Source: three-view drawing plus pictorial views. Frame: mm from the lowest corner of the part. Round coordinates to 2 decimals unless told otherwise and drop trailing zeros. Loops run counter-clockwise (first coordinate to the right, second up) from the corner with the lowest first, then second, coordinate; pieces in that order, holes last. Notation, with made-up numbers: (45.5, 85.25) -> (76.5, 85.25) arc R20 ccw to (76.5, 118.25) -> close; hole circle Ø7 at (46.25, -20). An arc over 180 degrees is marked (long way). Answer as a JSON object with one key per item and string values. Group by question number.
Item 1: Section query D-D on y = 3.3. Return loops of the section in (x, z).
Item 2: Section query C-C on x = 24. Return loops of the section in (y, z), and give its area (3 significant figures).
Item 3: Section query A-A on x = 70.5. Return loops of the section in (y, z).
Item 4: Section query B-B on z = 44. Return loops of the section in (x, y).
Item 5: Pin query (flat end, axial travel): pin 1 (10 mm diameter, centred on x = 38, z = 23.5, fed in from +Y); pin 2 (5.5 mm diameter, centred on x = 4, z = 44, fed in from -Y); pin 3 (0.9 mm diameter, centred on y = 3.5, z = 35, fed in from -X); pin 4 (1 mm diameter, centred on y = 3.5, z = 36, fed in from +X). Return the tip coordinate at first contact, or that it passes through.
Item 6: Material intervals for line 1 (X direction, y = 1.15, z = 44); line 2 (Y direction, x = 42.5, z = 30); line 3 (X direction, y = 3, z = 13), sorted ascending. Write a range as [from, to].
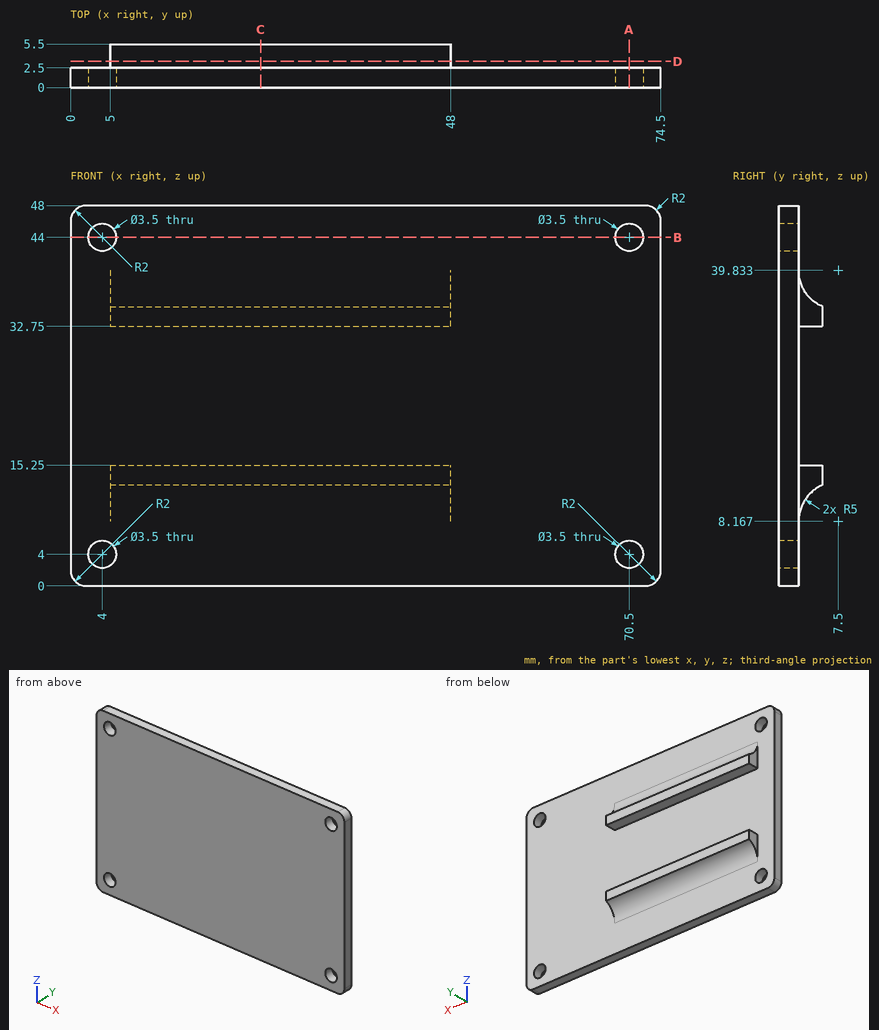
Solved:
{
 "1": {"outline": "(5, 10.88) -> (48, 10.88) -> (48, 15.25) -> (5, 15.25) -> close; (5, 32.75) -> (48, 32.75) -> (48, 37.12) -> (5, 37.12) -> close"},
 "2": {"outline": "(0, 0) -> (2.5, 0) -> (2.5, 8.17) arc R5 cw to (5.5, 12.75) -> (5.5, 15.25) -> (2.5, 15.25) -> (2.5, 32.75) -> (5.5, 32.75) -> (5.5, 35.25) arc R5 cw to (2.5, 39.83) -> (2.5, 48) -> (0, 48) -> close", "area": "143 mm²"},
 "3": {"outline": "(0, 0) -> (2.5, 0) -> (2.5, 2.25) -> (0, 2.25) -> close; (0, 5.75) -> (2.5, 5.75) -> (2.5, 42.25) -> (0, 42.25) -> close; (0, 45.75) -> (2.5, 45.75) -> (2.5, 48) -> (0, 48) -> close"},
 "4": {"outline": "(0, 0) -> (2.25, 0) -> (2.25, 2.5) -> (0, 2.5) -> close; (5.75, 0) -> (68.75, 0) -> (68.75, 2.5) -> (5.75, 2.5) -> close; (72.25, 0) -> (74.5, 0) -> (74.5, 2.5) -> (72.25, 2.5) -> close"},
 "5": {"pin 1": "y = 2.5", "pin 2": "y = 0", "pin 3": "x = 5", "pin 4": "x = 48"},
 "6": {"line 1": "[0, 2.25], [5.75, 68.75], [72.25, 74.5]", "line 2": "[0, 2.5]", "line 3": "[5, 48]"}
}
